For this review, use the dimensioned drawing (mm, ordinates from the lowest corner) and the shaded views. A direction names the side the tool comes from. Round coordinates to 2 decimals unless told otherwise and drop trailing zeros. Loops run counter-clockwise (first coordinate to the right, second up) from the corner with the lowest first, then second, coordinate; pieces in that order, holes last. Notation, with made-up numbers: M 2.5,23 L 29.5,23 A26 ccw 29.5,51 Z; hole C -9.75,73.25 d6. An arc over 180 degrees is marked long. Answer as a JSON object with one key per item and string values. Group by question number.
Item 1: To check wall thickness, follow line 1 (Y direction, x = 7.25, z = 8.5); line 2 (Y direction, x = 4.25, z = 10.25); line 3 (Z direction, x = 4.5, y = 9.5). State the ranges of each line that lie inside material, in increasing order.
Item 2: Tool access review of the marked faces 5 and 6: name each direction out of +Z, -Z, +X, -X, +Y, -Y from which nothing blocks a thin tool from reaching the whole face with its end or side.
Item 3: Consider section A-A (z = 10.5). Give the boundary of the cut face in (x, y) (3 decimals), and give its area (3 significant figures).
Item 4: Insertion check: P1, Ø1, axis at x = 2, y = 10.5, coming from the -Z side; P2, Ø4, axis at x = 6.5, z = 2.5, coming from the -Y side. Each pin has a flat end and moves straight along its axis. Give the tip position at first contact, or say it passes through.
Item 5: The part is to be moulded in two halves that separate along Y. For the marked faces 1, 2, 3 and 4, say which applies: +Y half, -Y half, draft (parallel to the pull), parting line (faces both ways), or undercut.
Item 6: Consider section B-B (x = 4). Give the boundary of the cut face in (y, z).
Item 7: Consider section C-C (y = 5). Give the boundary of the cut face in (x, z).
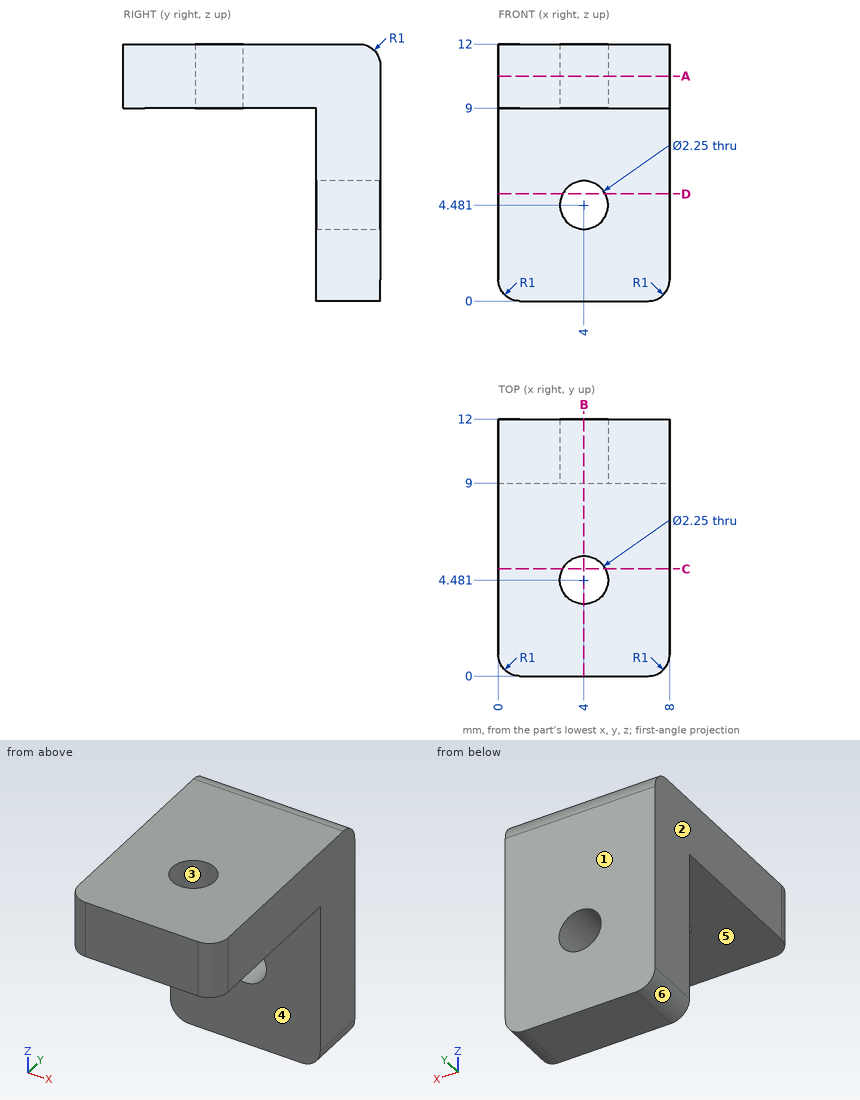
Geometry results:
{
 "1": {"line 1": "y = 9 to 12", "line 2": "y = 0 to 3.38, 5.58 to 12", "line 3": "z = 0 to 3.47, 5.49 to 12"},
 "2": {"face 5": "-Z, +X, -X, -Y", "face 6": "-Z, -X, +Y, -Y"},
 "3": {"outline": "M 0,1 A1 ccw 1,0 L 7,0 A1 ccw 8,1 L 8,12 L 0,12 Z; hole C 4,4.481 d2.25", "area": "91.6 mm^2"},
 "4": {"P1": "stops at z = 0", "P2": "stops at y = 9"},
 "5": {"face 1": "+Y half", "face 2": "draft", "face 3": "undercut", "face 4": "-Y half"},
 "6": {"outline": "M 0,9 L 3.36,9 L 3.36,12 L 0,12 Z; M 5.61,9 L 9,9 L 9,5.61 L 12,5.61 L 12,11 A1 ccw 11,12 L 5.61,12 Z; M 9,0 L 12,0 L 12,3.36 L 9,3.36 Z"},
 "7": {"outline": "M 0,9 L 3,9 L 3,12 L 0,12 Z; M 5,9 L 8,9 L 8,12 L 5,12 Z"}
}
